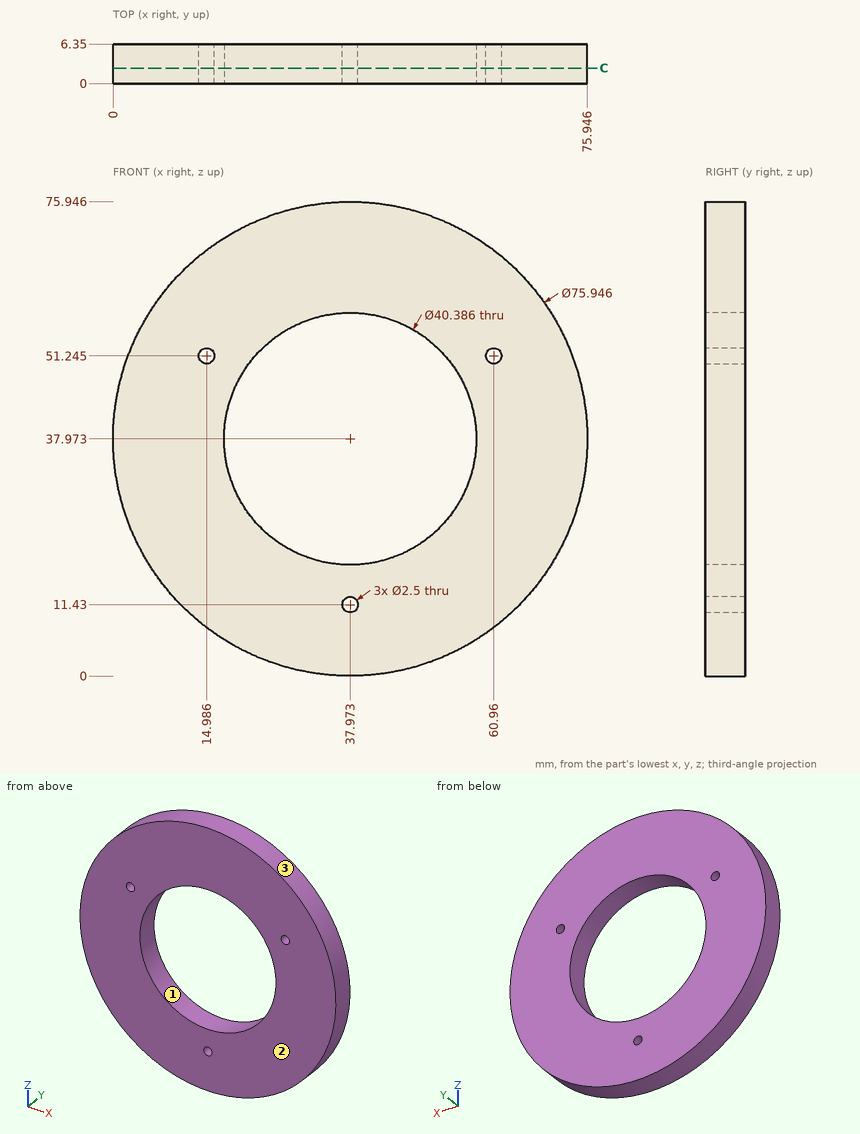
Job drawing, mm, ordinate dimensions from the low corner. One solid piece. Round coordinates to 2 decimals unless told otherwise and drop trailing zeros. Answer as a JSON object with one key per item and string values.
(1) Band-saw the part on C-C, the plane y = 2.5. Count the separate pieces of the cut face and the enclosed holes in it, then the cut area to 3 significant figures.
Reported:
{"separate pieces": "1", "enclosed holes": "4", "area": "3,230 mm^2"}
(2) Two-plate mould, pull along X, no slides. Class the marked faces 1, 2 and 3: +X half, -X half, draft (parallel to the pull), parting line (faces both ways), or undercut.
Reported:
{"face 1": "undercut", "face 2": "draft", "face 3": "parting line"}
(3) Probe probe 1 along X at (y, z) = (5.25, 37.5) (1 decimal); probe 2 along X at (y, z) = (3, 50.5) (1 decimal); probe 3 along X at (y, z) = (4, 35) (1 decimal). List the from-to ranges inside material, lowest first. Write a range as [from, to].
Reported:
{"probe 1": "x = [0, 17.8], [58.2, 75.9]", "probe 2": "x = [2.1, 14], [16, 22.1], [53.8, 60], [62, 73.8]", "probe 3": "x = [0.1, 18], [57.9, 75.8]"}
(4) Pin check, flat tips, straight feed: P1, Ø3, axis at x = 64.5, y = 4.5, coming from the +Z side; P2, Ø1.5, axis at x = 16.5, y = 3, coming from the +Z side. Stop position of each tip, or through.
Reported:
{"P1": "stops at z = 66.53", "P2": "stops at z = 69.79"}
